Geometry: final body of the model. Coordinates: model frame, mm. A direction names the side the tool comes from. Round coordinates to 2 decimals unless told otherwise and drop trailing zeros. Loops run counter-clockwise (first coordinate to the right, second up) from the corner with the lowest first, then second, coordinate; pieces in that order, holes last. Notation, with made-up numbers: M 1.5,14 L 26.5,14 A19 ccw 26.5,36 Z; hole C -34.5,48.5 d10. An arc over 180 degrees is marked long. Answer as a JSON object with one key per item and string values.
from build123d import *

# Parameters (mm, degrees)
SKETCH_R             = 2.125
SKETCH_R_2           = 2.5
PAD_DEPTH            = 6
SKETCH001_R          = 2.125
PAD001_DEPTH         = 10
SKETCH002_W          = 1
SKETCH002_H          = 20
POCKET_DEPTH         = 10.001
SKETCH003_R          = 1.75
POCKET001_DEPTH      = 10.001
POCKET001_DEPTH_BACK = -10.001
POCKET002_DEPTH      = 3


with BuildPart() as part:
    # Sketch → Pad (new body)
    with BuildSketch(Plane.XY):
        Polygon((-5, 40), (5, 40), (5, 20), (10, 20), (10, 0), (-10, 0), (-10, 20), (-5, 20), align=None)
        with Locations((0, 30)):
            Circle(SKETCH_R, mode=Mode.SUBTRACT)
        with Locations((0, 10)):
            Circle(SKETCH_R_2, mode=Mode.SUBTRACT)
    extrude(amount=PAD_DEPTH)

    # Sketch001 → Pad001 (join)
    with BuildSketch(Plane.XY):
        with BuildLine():
            ThreePointArc((-4, 30), (0, 26), (4, 30))
            Line((4, 30), (5, 30))
            Line((5, 30), (5, 40))
            Line((-5, 40), (5, 40))
            Line((-5, 30), (-5, 40))
            Line((-4, 30), (-5, 30))
        make_face()
        with Locations((0, 30)):
            Circle(SKETCH001_R, mode=Mode.SUBTRACT)
    extrude(amount=PAD001_DEPTH)

    # Sketch002 → Pocket (cut, through all)
    with BuildSketch(Plane.XY):
        with Locations((0, 40)):
            Rectangle(SKETCH002_W, SKETCH002_H)
    extrude(amount=POCKET_DEPTH, mode=Mode.SUBTRACT)

    # Sketch003 → Pocket001 (cut, two sides)
    with BuildSketch(Plane.YZ) as pocket001_sk:
        with Locations((36, 5)):
            Circle(SKETCH003_R)
    extrude(amount=-POCKET001_DEPTH, mode=Mode.SUBTRACT)
    extrude(pocket001_sk.sketch, amount=-POCKET001_DEPTH_BACK, mode=Mode.SUBTRACT)

    # Sketch004 (on Face14 of Pocket001) → Pocket002 (cut)
    with BuildSketch(Plane.YZ.offset(5)):
        Polygon((39.031089, 3.25), (39.031089, 6.75), (36, 8.5), (32.968911, 6.75), (32.968911, 3.25), (36, 1.5), align=None)
    extrude(amount=-POCKET002_DEPTH, mode=Mode.SUBTRACT)


solid = part.part
1) Section query B-B (z = 5). Return the cut outline in (x, y) (3 decimals), and give its area (3 significant figures).
Results:
{"outline": "M -10,0 L 10,0 L 10,20 L 5,20 L 5,32.969 L 2,32.969 L 2,34.25 L 0.5,34.25 L 0.5,32.065 A2.125 cw long -0.5,32.065 L -0.5,34.25 L -5,34.25 L -5,20 L -10,20 Z; M -5,37.75 L -0.5,37.75 L -0.5,40 L -5,40 Z; M 0.5,37.75 L 2,37.75 L 2,39.031 L 5,39.031 L 5,40 L 0.5,40 Z; hole C 0,10 d5", "area": "519 mm2"}
2) Reachability of faces 1 (the flat face through (7, 20, 3)), 2 (the flat face through (4.5, 30, 8)), 3 (the flat face through (-0.5, 34, 5)), 4 (the flat face through (3.52, 37.49, 2.36)) from +Z, -Z, +X, -X, +Y, -Y: full face, straight path, thin tool, end or side. Return the list, or none.
Results:
{"face 1": "+Z, -Z, +X, +Y", "face 2": "+Z, +X, -Y", "face 3": "+Z, -Z, +Y", "face 4": "+X"}
3) Pin query (flat end, axial travel): P1, Ø0.8, axis at x = -4.5, z = 8, coming from the -Y side; P2, Ø10, axis at x = -0.5, y = 16, coming from the +Z side; P3, Ø4.5, axis at y = 36, z = 5, coming from the +X side; P4, Ø4, axis at x = 0, y = 10, coming from the -Z side. Return the tip coordinate at first contact, or that it passes through.
Results:
{"P1": "y = 30", "P2": "z = 6", "P3": "x = 2", "P4": "through"}
4) Section query D-D (y = 35). Return the cut outline in (x, z), and give its area (3 significant figures).
Results:
{"outline": "M -5,0 L -0.5,0 L -0.5,3.56 L -5,3.56 Z; M -5,6.44 L -0.5,6.44 L -0.5,10 L -5,10 Z; M 0.5,0 L 5,0 L 5,2.08 L 2,2.08 L 2,3.56 L 0.5,3.56 Z; M 0.5,6.44 L 2,6.44 L 2,7.92 L 5,7.92 L 5,10 L 0.5,10 Z", "area": "55.2 mm2"}
5) Section query C-C (x = 0). Return the cut outline in (y, z) (3 decimals), and give its area (3 significant figures).
Results:
{"outline": "M 0,0 L 7.5,0 L 7.5,6 L 0,6 Z; M 12.5,0 L 27.875,0 L 27.875,10 L 26,10 L 26,6 L 12.5,6 Z", "area": "145 mm2"}
6) Pull-direction query (Z, two-part tool) for faces 5 (the flat face through (4, 39.031, 5)), 6 (the flat face through (-3, 40, 5)), 7 (the flat face through (0, 16, 0)), 8 (the flat face through (3.52, 34.51, 7.64)); classes: +Z half, -Z half, draft (parallel to the pull), parting line (faces both ways), or undercut.
Results:
{"face 5": "undercut", "face 6": "draft", "face 7": "-Z half", "face 8": "undercut"}
7) Section query A-A (y = 12). Return the cut outline in (x, z), and give its area (3 significant figures).
Results:
{"outline": "M -10,0 L -1.5,0 L -1.5,6 L -10,6 Z; M 1.5,0 L 10,0 L 10,6 L 1.5,6 Z", "area": "102 mm2"}
8) Ray query, line 1 (Z direction, x = -2.6, y = 36); line 2 (X direction, y = 30, z = 3.5) (3 decimals); line 3 (Y direction, x = 1.5, z = 2). Return the intervals inside material, ascending.
Results:
{"line 1": "0 to 3.25, 6.75 to 10", "line 2": "-5 to -2.125, 2.125 to 5", "line 3": "0 to 8, 12 to 28.49, 31.51 to 40"}
